```python
from build123d import *

# Parameters (mm, degrees)
SKETCH2_R           = 5
BOSS_EXTRUDE1_DEPTH = 17.5
SKETCH3_R           = 5
CUT_EXTRUDE1_DEPTH  = 52.326162919


with BuildPart() as part:
    # Sketch2 → Boss-Extrude1 (new body)
    with BuildSketch(Plane(origin=(0, 0, 0), x_dir=(1, 0, 0), z_dir=(0, 1, 0))):
        with BuildLine():
            Line((-8.75, -7.5), (-8.75, 20))
            ThreePointArc((-8.75, 20), (0, 28.75), (8.75, 20))
            Line((8.75, 20), (8.75, -7.5))
            ThreePointArc((8.75, -7.5), (10.946699141, -12.803300859), (16.25, -15))
            Line((16.25, -15), (30, -15))
            Line((30, -15), (30, -20))
            Line((30, -20), (-30, -20))
            Line((-30, -20), (-30, -15))
            Line((-30, -15), (-16.25, -15))
            ThreePointArc((-16.25, -15), (-10.946699141, -12.803300859), (-8.75, -7.5))
        make_face()
        with Locations(Location((0, 20, 0), (0, 0, 270))):
            Circle(SKETCH2_R, mode=Mode.SUBTRACT)
    extrude(amount=BOSS_EXTRUDE1_DEPTH)

    # Sketch3 → Cut-Extrude1 (cut, through all)
    with BuildSketch(Plane.ZY.offset(8.75)):
        with Locations((-6.25, 8.75)):
            Circle(SKETCH3_R)
    extrude(amount=-CUT_EXTRUDE1_DEPTH, mode=Mode.SUBTRACT)


solid = part.part
```
Check sheet for the modelled part. Datum: model origin and axes. Units: mm. A direction names the side the tool comes from. Give positions to 0.01 mm unless a question says otherwise; leave off trailing zeros. Order: outer loops, then holes, each group sorted by start corner. A loop starts at its lowest first (then second) coordinate and runs counter-clockwise, first axis right, second up. Notation, with made-up numbers: M 5.25,-9.75 L 31.25,-9.75 A26 ccw 31.25,17.25 Z; hole C 38,16 d10. An arc over 180 degrees is marked long. Answer in a Markdown table with one row per item.
1) Cross-section at D-D, the plane y = 2.25. Enter the section's corners in (x, z).
Filled sheet:
| item | result |
|---|---|
| outline | M -30,15 L -16.25,15 A7.5 cw -8.75,7.5 L -8.75,-20 A8.75 ccw 8.75,-20 L 8.75,7.5 A7.5 cw 16.25,15 L 30,15 L 30,20 L -30,20 Z; hole C 0,-20 d10 |
2) Access from +Z, -Z, +X, -X, +Y, -Y to the whole of each face (thin tool, end or side, straight path). Record for faces 5 (the flat face through (-23, 9, 15)), 6 (the flat face through (23, 9, 15)), 7 (the flat face through (-2, 0, 3)).
Filled sheet:
| item | result |
|---|---|
| face 5 | -Z, -X, +Y, -Y |
| face 6 | -Z, +X, +Y, -Y |
| face 7 | +Z, -Z, +X, -X, -Y |
3) Cross-section at B-B, the plane y = 8.75. Enter the section's corners in (x, z), plus the area to 3 significant figures.
Filled sheet:
| item | result |
|---|---|
| outline | M -30,15 L -16.25,15 A7.5 cw -8.75,7.5 L -8.75,-1.25 L 8.75,-1.25 L 8.75,7.5 A7.5 cw 16.25,15 L 30,15 L 30,20 L -30,20 Z; M -8.75,-20 A8.75 ccw 8.75,-20 L 8.75,-11.25 L -8.75,-11.25 Z; hole C 0,-20 d10 |
| area | 803 mm2 |
4) Cross-section at C-C, the plane z = -6.25. Enter the section's corners in (x, y), plus the area to 3 significant figures.
Filled sheet:
| item | result |
|---|---|
| outline | M -8.75,0 L 8.75,0 L 8.75,3.75 L -8.75,3.75 Z; M -8.75,13.75 L 8.75,13.75 L 8.75,17.5 L -8.75,17.5 Z |
| area | 131 mm2 |
5) Release check for a two-part mould opening along Z. For faces 1 (the flat face through (0, 9, 20)), 2 (the cylindrical face through (10.889, 8.628, 12.745)), 3 (the cylindrical face through (0, 9, -25)), 4 (the flat face through (-8.75, 4.7, -3)) record: +Z half, -Z half, draft (parallel to the pull), parting line (faces both ways), or undercut.
Filled sheet:
| item | result |
|---|---|
| face 1 | +Z half |
| face 2 | -Z half |
| face 3 | undercut |
| face 4 | draft |
6) Gauge pin test, flat ends, axial feed: P1, Ø5, axis at y = 6, z = -2, coming from the +X side; P2, Ø9, axis at y = 9, z = -8.5, coming from the -X side; P3, Ø9, axis at x = 0, z = -20, coming from the +Y side; P4, Ø4, axis at x = -22, y = 7, coming from the -Z side. Record the tip position at first contact, or that the pin passes through.
Filled sheet:
| item | result |
|---|---|
| P1 | stops at x = 8.75 |
| P2 | stops at x = -8.75 |
| P3 | passes through |
| P4 | stops at z = 15 |
7) Cross-section at A-A, the plane x = 0. Enter the section's corners in (y, z), plus the area to 3 significant figures.
Filled sheet:
| item | result |
|---|---|
| outline | M 0,-28.75 L 17.5,-28.75 L 17.5,-25 L 0,-25 Z; M 0,-15 L 17.5,-15 L 17.5,20 L 0,20 Z; hole C 8.75,-6.25 d10 |
| area | 600 mm2 |
8) Thickness scan on L1, parallel to Y at x = -4, z = -6.25; L2, parallel to X at y = 9.5, z = -20; L3, parallel to Z at x = -3, y = 8. Record the ranges inside material, lowest first. Write a range as [from, to].
Filled sheet:
| item | result |
|---|---|
| L1 | y = [0, 3.75], [13.75, 17.5] |
| L2 | x = [-8.75, -5], [5, 8.75] |
| L3 | z = [-28.22, -24], [-16, -11.19], [-1.31, 20] |
